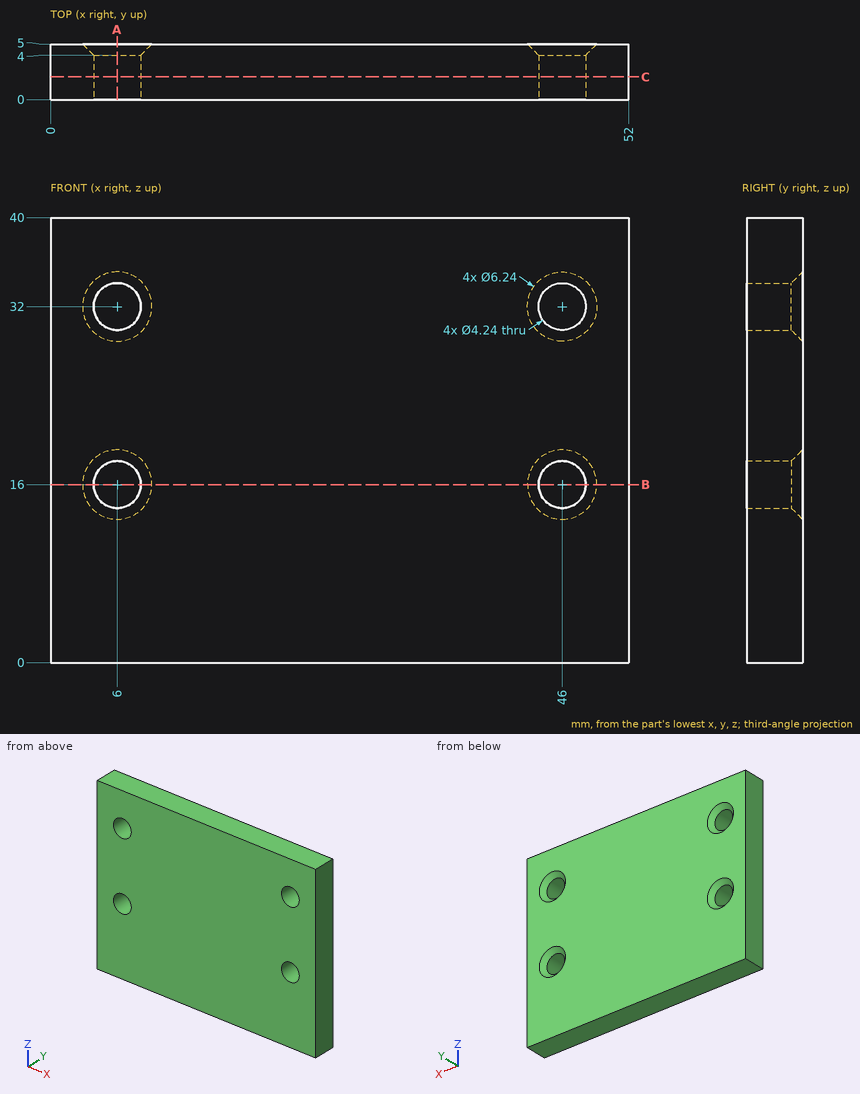
The figure shows three views and two pictorial views of one solid part (mm, origin at its lowest corner). Answer the questions. Round coordinates to 2 decimals unless told otherwise and drop trailing zeros. Write each loop counter-clockwise with the first axis right and the second up, starting at its lowest first coordinate (ties: lowest second). Pieces come first, ordered by that corner, then holes. Notation, with made-up numbers: M -5.5,-23.75 L 12.5,-23.75 A11 ccw 12.5,-18.75 Z; hole C 38.5,77.5 d4. An arc over 180 degrees is marked long. Use a Markdown table: item, result.
1) Straight lines are drawn through the part: line 1 along X through (y, z) = (1.9, 16); line 2 along Z through (x, y) = (46, 2.75); line 3 along X through (y, z) = (2.05, 33.5). For each, find the intervals that lie inside material, in ascending order. Write a range as [from, to].
Answers follow:
| item | result |
|---|---|
| line 1 | x = [0, 3.88], [8.12, 43.88], [48.12, 52] |
| line 2 | z = [0, 13.88], [18.12, 29.88], [34.12, 40] |
| line 3 | x = [0, 4.5], [7.5, 44.5], [47.5, 52] |
2) A flat-ended cylindrical pin translates along its axis: pin 1 (2.5 mm diameter, centred on x = 6, z = 16, fed in from +Y). Find the tip coordinate at first contact, or state that the pin passes through.
Answers follow:
| item | result |
|---|---|
| pin 1 | passes through |
3) The part is cut by section A-A (x = 6). Write down the section's boundary in (y, z), plus the area to 3 significant figures.
Answers follow:
| item | result |
|---|---|
| outline | M 0,0 L 5,0 L 5,12.88 L 4,13.88 L 0,13.88 Z; M 0,18.12 L 4,18.12 L 5,19.12 L 5,28.88 L 4,29.88 L 0,29.88 Z; M 0,34.12 L 4,34.12 L 5,35.12 L 5,40 L 0,40 Z |
| area | 156 mm2 |
4) The part is cut by section C-C (y = 2.05). Write down the section's boundary in (x, z).
Answers follow:
| item | result |
|---|---|
| outline | M 0,0 L 52,0 L 52,40 L 0,40 Z; hole C 6,16 d4.24; hole C 6,32 d4.24; hole C 46,16 d4.24; hole C 46,32 d4.24 |
5) The part is cut by section B-B (z = 16). Write down the section's boundary in (x, y).
Answers follow:
| item | result |
|---|---|
| outline | M 0,0 L 3.88,0 L 3.88,4 L 2.88,5 L 0,5 Z; M 8.12,0 L 43.88,0 L 43.88,4 L 42.88,5 L 9.12,5 L 8.12,4 Z; M 48.12,0 L 52,0 L 52,5 L 49.12,5 L 48.12,4 Z |
